Read the model definition and answer for the solid it produces. Units are mm, in the model's axes. A direction names the side the tool comes from. Coordinates: 2 decimals unless noted, no trailing zeros. Write each loop counter-clockwise with the first axis right and the second up, starting at its lowest first coordinate (ties: lowest second). Pieces come first, ordered by that corner, then holes. Notation, with made-up numbers: (16.5, 19) -> (50.5, 19) arc R26 ccw to (50.5, 55) -> close; hole circle Ø10 at (-17.75, 86). An arc over 180 degrees is marked (long way). One line per item, written item: value. Start each with the question number.
Solid Edge part; units mm, degrees
sketch "Sketch1" plane through (0, 0, 0) normal (0, -1, 0) x (1, 0, 0)
  line L0 (21.2, 4.4667) -> (41.2, 4.4667)
  line L1 (41.2, 4.4667) -> (41.2, 44.4667)
  line L2 (41.2, 44.4667) -> (21.2, 44.4667)
  line L3 (21.2, 44.4667) -> (21.2, 4.4667)
  dimension "D1" = 21.2
  dimension "D2" = 41.2
extrude "Protrusion1" add sketch "Sketch1" against normal blind 15
sketch "Sketch2" plane through (31.2, 0, 24.4667) normal (0, -1, 0) x (1, 0, 0)
  circle A0 centre (0, 10) radius 6.75
extrude "ExtrudedCutout_1" cut sketch "Sketch2" against normal blind 10
sketch "Sketch3" plane through (21.2, 7.5, 24.4667) normal (-1, 0, 0) x (0, -1, 0)
  line L0 (7.5, 13) -> (2.5, 13)
  arc A0 (2.5, 6.5) -> (2.5, 13) centre (2.5, 9.75) cw
  line L1 (7.5, 6.5) -> (2.5, 6.5)
  line L2 (7.5, 13) -> (7.5, 6.5)
  dimension "D1" = 7.5
  dimension "D2" = 7.5
  dimension "D3" = 7.5
extrude "Cutout1" cut sketch "Sketch3" against normal through all
sketch "Sketch4" plane through (31.2, 15, 24.4667) normal (0, 1, 0) x (-1, 0, 0)
  line L0 (-10, 20) -> (-9, 20)
  line L1 (-9, 20) -> (-9, -20)
  line L2 (-9, -20) -> (-10, -20)
  line L3 (-10, -20) -> (-10, 20)
  dimension "D1" = 10
extrude "Cutout2" cut sketch "Sketch4" against normal through all
sketch "Sketch5" plane through (28.2, 7.5, 4.4667) normal (0, 0, -1) x (1, 0, 0)
  line L0 (6.5, 7.5) -> (6.5, 2.5)
  arc A0 (6.5, 2.5) -> (0, 2.5) centre (3.25, 2.5) cw
  line L1 (0, 2.5) -> (0, 7.5)
  line L2 (6.5, 7.5) -> (0, 7.5)
  dimension "D1" = 6.5
extrude "Cutout3" cut sketch "Sketch5" against normal up to next
sketch "Sketch6" plane through (28.2, 15, 24.4667) normal (0, 1, 0) x (-1, 0, 0)
  line L0 (-12, -20) -> (7, -20)
  line L1 (7, -20) -> (7, -1)
  line L2 (7, -1) -> (-12, -1)
  line L3 (-12, -1) -> (-12, -20)
  dimension "D1" = 7
extrude "Cutout4" cut sketch "Sketch6" against normal up to next
sketch "Sketch7" plane through (28.2, 15, 33.9667) normal (0, 1, 0) x (-1, 0, 0)
  line L0 (-39.04, 20.5) -> (-39.04, -19.5)
  line L1 (-39.04, -19.5) -> (50.96, -19.5)
  line L2 (50.96, 20.5) -> (50.96, -19.5)
  line L3 (-39.04, 20.5) -> (50.96, 20.5)
  dimension "D1" = 39.04
  dimension "D2" = 39.04
  dimension "D3" = 50.96
extrude "ExtrudedProtrusion_2" add sketch "Sketch7" along normal blind 3
sketch "Sketch8" plane through (19.24, 18, 34.4667) normal (0, 1, 0) x (-1, 0, 0)
  circle A0 centre (-43, 15) radius 1.65
  circle A1 centre (37, -15) radius 1.65
  dimension "D1" = 43
extrude "Cutout5" cut sketch "Sketch8" against normal through all
sketch "Sketch9" plane through (19.24, 18, 34.4667) normal (0, 1, 0) x (-1, 0, 0)
  circle A0 centre (-43, 15) radius 3.55
  circle A1 centre (37, -15) radius 3.55
extrude "ExtrudedCutout_9" cut sketch "Sketch9" against normal blind 0.5
1. A tool of negligible diameter and unlimited length cuts with its end or side. For faces 5 (the face through (34.7, 2, 26)), 6 (the face through (26.2, 6, 39)), 7 (the face through (39, 2, 37.467)), 8 (the face through (31, 7, 44.467)), from which of +Z, -Z, +X, -X, +Y, -Y can it reach the whole face along a straight path? Write none if from no direction.
2. A cutting plane is placed at C-C on x = 31.45. Give the vertices of the cut face in (y, z).
3. A cutting plane is placed at D-D on x = 51.5. Give the vertices of the cut face in (y, z), then the cut area to 3 significant figures.
4. A cutting plane is placed at B-B on y = 13. Give the vertices of the cut face in (x, z), then the cut area to 3 significant figures.
5. Find the intervals of material crossed by probe 1 along Z at (x, y) = (-17.76, 17.75); probe 2 along X at (y, z) = (5.25, 25.5); probe 3 along Z at (x, y) = (62.24, 17.85), in increasing order. Write a range as from..to.
6. Given pin 1 (2 mm diameter, centred on x = 62.24, z = 49.47, fed in from -Y); pin 2 (8 mm diameter, centred on x = 62.24, z = 49.47, fed in from +Y); pin 3 (1.5 mm diameter, centred on x = 38, y = 3.5, fed in from -Z); pin 4 (5.5 mm diameter, centred on x = -17.76, z = 19.47, fed in from +Y), each flat-ended and moving along its own axis, determine where each tip first touches the part or whether it passes through.
7. For a pull along Z with two mould halves and no side action, classify faces 1 (the face through (31, 9, 23.467)), 2 (the face through (65.06, 17.75, 47.31)), 3 (the face through (40.2, 9, 34)), 4 (the face through (38.92, 8.25, 34.29)) as +Z half, -Z half, draft (parallel to the pull), parting line (faces both ways), or undercut.
8. A cutting plane is placed at A-A on x = 62.24. Give the vertices of the cut face in (y, z), then the cut area to 3 significant figures.
Derived:
1. face 5: -Z, -Y
1. face 6: -Y
1. face 7: +X, -X, -Y
1. face 8: +Z, +X, -X, -Y
2. outline: (0, 41.21) -> (10, 41.21) -> (10, 27.72) -> (8.25, 27.72) -> (8.25, 23.47) -> (15, 23.47) -> (15, 14.47) -> (18, 14.47) -> (18, 54.47) -> (15, 54.47) -> (15, 44.47) -> (0, 44.47) -> close
3. outline: (15, 14.47) -> (18, 14.47) -> (18, 54.47) -> (15, 54.47) -> close
3. area: 120 mm2
4. outline: (21.2, 23.47) -> (40.2, 23.47) -> (40.2, 44.47) -> (21.2, 44.47) -> close
4. area: 399 mm2
5. probe 1: z = 14.47..15.92, 23.02..54.47
5. probe 2: x = 21.2..28.21, 34.69..40.2
5. probe 3: z = 14.47..45.92, 53.02..54.47
6. pin 1: passes through
6. pin 2: stops at y = 18
6. pin 3: stops at z = 23.47
6. pin 4: stops at y = 17.5
7. face 1: -Z half
7. face 2: undercut
7. face 3: draft
7. face 4: undercut
8. outline: (15, 14.47) -> (18, 14.47) -> (18, 45.92) -> (17.5, 45.92) -> (17.5, 47.82) -> (15, 47.82) -> close; (15, 51.12) -> (17.5, 51.12) -> (17.5, 53.02) -> (18, 53.02) -> (18, 54.47) -> (15, 54.47) -> close
8. area: 108 mm2
